Study the drawing (mm; zero at the part's minimum x, y, z) and answer. A direction names the side the tool comes from. Coordinates: 2 decimals unless noted, no trailing zeros. Order: outer loops, then holes, each group sorted by start corner. A loop starts at its lowest first (then second) coordinate and runs counter-clockwise, first axis right, second up. Notation, with made-up numbers: M -4,28 L 42,28 A22 cw 42,64 Z; hole C 21.5,50.25 d2. An arc over 180 degrees is marked long. Put each result on its own line as item: value.
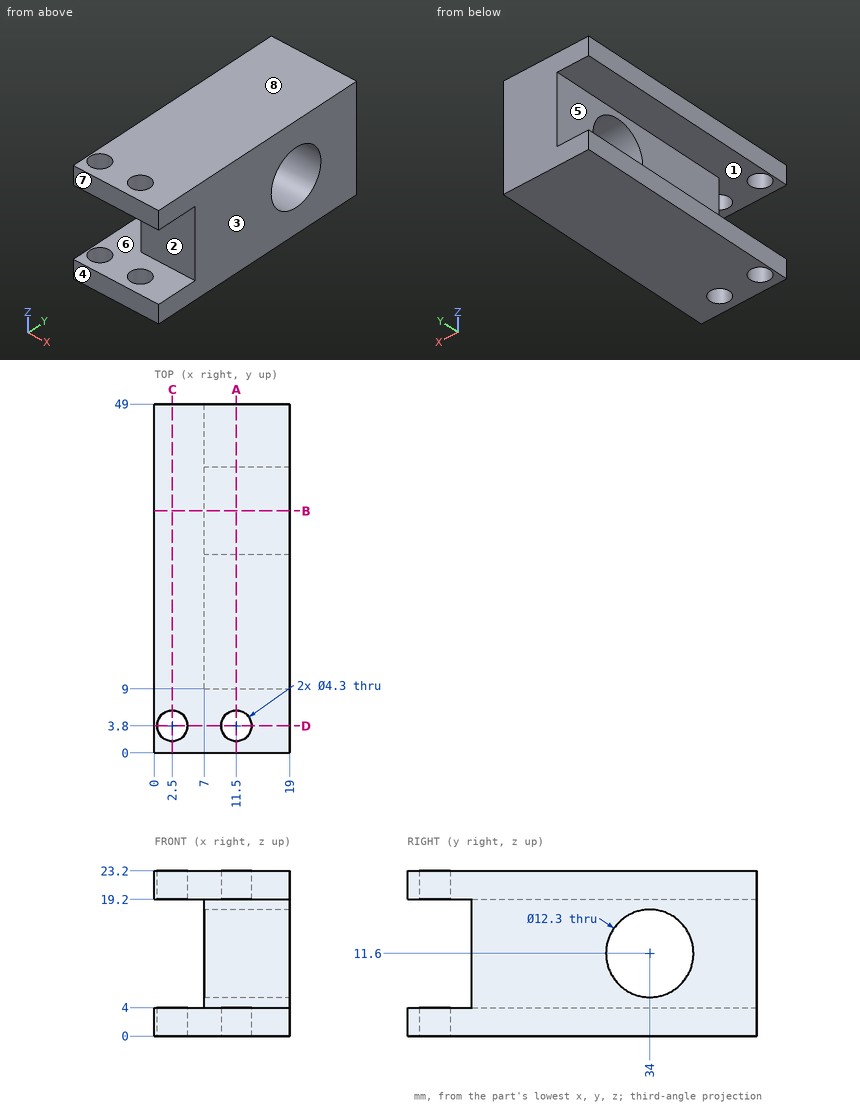
Q1. Given pin 1 (11 mm diameter, centred on y = 34, z = 11.6, fed in from +X); pin 2 (12 mm diameter, centred on y = 40, z = 11, fed in from -X), each flat-ended and moving along its own axis, determine where each tip first touches the part or whether it passes through.
Answers below:
pin 1: passes through
pin 2: stops at x = 7
Q2. Find section C-C on x = 2.5. Write down the section's boundary in (y, z).
Answers below:
outline: M 0,0 L 1.65,0 L 1.65,4 L 0,4 Z; M 0,19.2 L 1.65,19.2 L 1.65,23.2 L 0,23.2 Z; M 5.95,0 L 49,0 L 49,4 L 5.95,4 Z; M 5.95,19.2 L 49,19.2 L 49,23.2 L 5.95,23.2 Z
Q3. Find section A-A on x = 11.5. Write down the section's boundary in (y, z).
Answers below:
outline: M 0,0 L 1.65,0 L 1.65,4 L 0,4 Z; M 0,19.2 L 1.65,19.2 L 1.65,23.2 L 0,23.2 Z; M 5.95,0 L 49,0 L 49,23.2 L 5.95,23.2 L 5.95,19.2 L 9,19.2 L 9,4 L 5.95,4 Z; hole C 34,11.6 d12.3
Q4. A tool of negligible diameter and unlimited length cuts with its end or side. For the marked faces 1, 2, 3, 4 and 5, from which of +Z, -Z, +X, -X, +Y, -Y can it reach the whole face along a straight path? Write none if from no direction.
Answers below:
face 1: -X, -Y
face 2: +X, -X, -Y
face 3: +Z, -Z, +X, +Y, -Y
face 4: +Z, -Z, +X, -X, -Y
face 5: -X, +Y, -Y
Q5. Consider line 1 along X through (y, z) = (3.8, 1.55); line 2 along Z through (x, y) = (3.5, 22); line 3 along Y through (x, z) = (14, 11.6). Determine where each line is inside the solid, lowest interval first.
Answers below:
line 1: x = 0 to 0.35, 4.65 to 9.35, 13.65 to 19
line 2: z = 0 to 4, 19.2 to 23.2
line 3: y = 9 to 27.85, 40.15 to 49
Q6. For a pull along Z with two mould halves and no side action, classify the marked faces 6, 7 and 8 as +Z half, -Z half, draft (parallel to the pull), parting line (faces both ways), or undercut.
Answers below:
face 6: undercut
face 7: draft
face 8: +Z half
Q7. Find section B-B on y = 34. Write down the section's boundary in (x, z), plus the area to 3 significant figures.
Answers below:
outline: M 0,0 L 19,0 L 19,5.45 L 7,5.45 L 7,4 L 0,4 Z; M 0,19.2 L 7,19.2 L 7,17.75 L 19,17.75 L 19,23.2 L 0,23.2 Z
area: 187 mm^2
Q8. Find section D-D on y = 3.8. Write down the section's boundary in (x, z), plus the area to 3 significant figures.
Answers below:
outline: M 0,0 L 0.35,0 L 0.35,4 L 0,4 Z; M 0,19.2 L 0.35,19.2 L 0.35,23.2 L 0,23.2 Z; M 4.65,0 L 9.35,0 L 9.35,4 L 4.65,4 Z; M 4.65,19.2 L 9.35,19.2 L 9.35,23.2 L 4.65,23.2 Z; M 13.65,0 L 19,0 L 19,4 L 13.65,4 Z; M 13.65,19.2 L 19,19.2 L 19,23.2 L 13.65,23.2 Z
area: 83.2 mm^2
